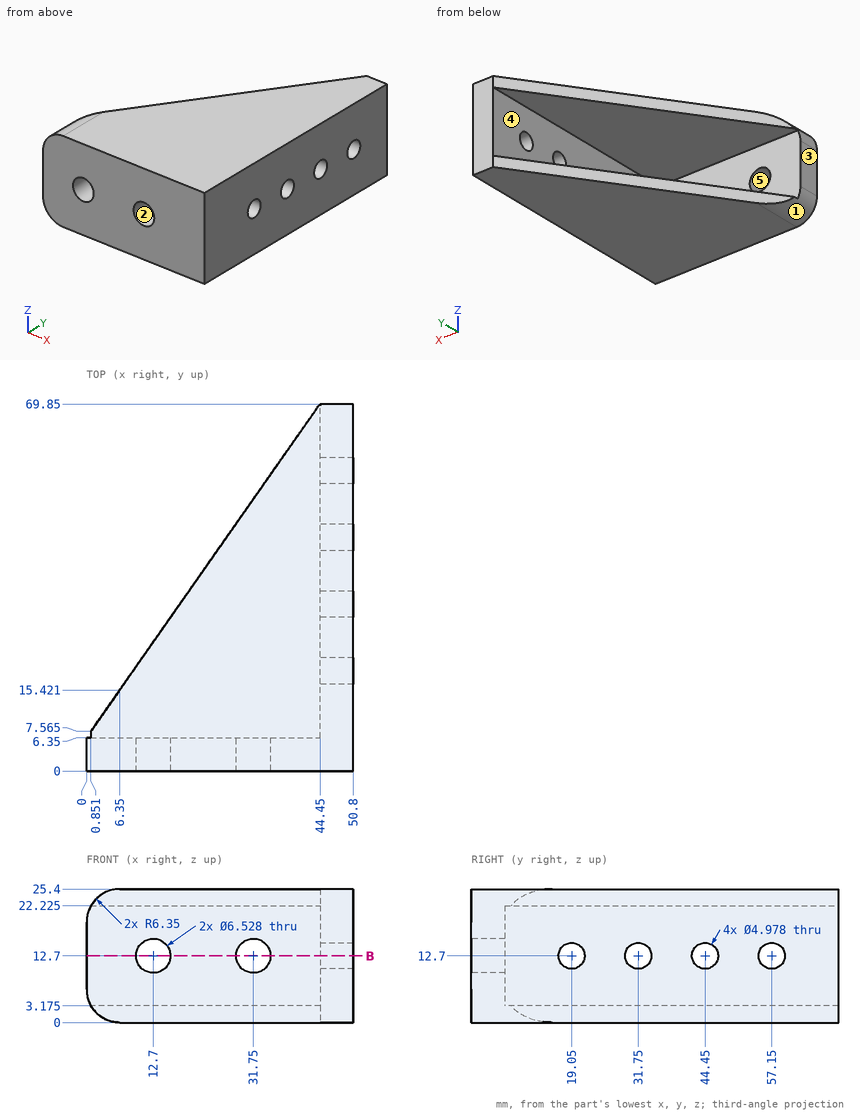
Here's the drawing with two shaded views (mm, measured from the low corner). I have some questions. A direction names the side the tool comes from. Coordinates: 2 decimals unless noted, no trailing zeros. Answer as CSV lines item,"result". Start each with the question number.
1) For the marked faces 4 and 5, which set-ups out of +Z, -Z, +X, -X, +Y, -Y let a thin tool reach every point of the face, with its end or its side?
2) For P1, Ø8, axis at y = 19.05, z = 12.7, coming from the +X side; P2, Ø9.5, axis at x = 18, z = 9, coming from the +Y side; P3, Ø5.5, axis at y = 31, z = 11, coming from the -X side, each with a flat end and sliding along its axis, tell me the tip position at first contact or that it passes through.
3) Please list where these lines run through material, in increasing order: line 1 (Y direction, x = 46, z = 12.7); line 2 (Z direction, x = 36.5, y = 57) (1 decimal); line 3 (Z direction, x = 12.7, y = 2.25). Write a range as from..to.
4) We'd pull the mould along Z, two halves only. Please class the marked faces 1, 2 and 3: +Z half, -Z half, draft (parallel to the pull), parting line (faces both ways), or undercut.
5) I want a section at B-B, the plane z = 12.7. Give the number of separate pieces and of enclosed holes in the cut face.
Data:
1,face 4,"-X, +Y"
1,face 5,"+Y, -Y"
2,P1,"stops at x = 50.8"
2,P2,"stops at y = 6.35"
2,P3,"stops at x = 44.45"
3,line 1,"y = 0..16.56, 21.54..29.26, 34.24..41.96, 46.94..54.66, 59.64..69.85"
3,line 2,"z = 0..3.2, 22.2..25.4"
3,line 3,"z = 0..9.44, 15.96..25.4"
4,face 1,"-Z half"
4,face 2,"undercut"
4,face 3,"draft"
5,separate pieces,"7"
5,enclosed holes,"0"
